```python
from build123d import *

# Parameters (mm, degrees)
BOSS_EXTRUDE1_DEPTH = 11
CUT_EXTRUDE1_DEPTH  = 7
SKETCH4_R           = 1.6
CUT_EXTRUDE2_DEPTH  = 19.607794066
SKETCH5_R           = 1.25
CUT_EXTRUDE3_DEPTH  = 21.451161336
CUT_EXTRUDE4_DEPTH  = 21.451161336
CUT_EXTRUDE5_DEPTH  = 5.8
SKETCH9_W           = 6.962435565
SKETCH9_H           = 4.2
CUT_EXTRUDE6_DEPTH  = 5.8
BOSS_EXTRUDE3_START = 0.2
BOSS_EXTRUDE3_DEPTH = 0.2
BOSS_EXTRUDE4_DEPTH = 7.3
CUT_EXTRUDE7_DEPTH  = 1.6


with BuildPart() as part:
    # Sketch1 → Boss-Extrude1 (new body)
    with BuildSketch(Plane.XY):
        Polygon((-8.5, 0), (8.5, 0), (8.5, 9), (7.5, 9), (7.5, 15), (-7.5, 15), (-7.5, 9), (-8.5, 9), align=None)
    extrude(amount=BOSS_EXTRUDE1_DEPTH)

    # Sketch2 → Cut-Extrude1 (cut)
    with BuildSketch(Plane.XY.offset(11)):
        with BuildLine():
            Line((3, 18), (3, 12))
            ThreePointArc((3, 12), (0, 9), (-3, 12))
            Line((-3, 12), (-3, 18))
            ThreePointArc((-3, 18), (0, 21), (3, 18))
        make_face()
    extrude(amount=-CUT_EXTRUDE1_DEPTH, mode=Mode.SUBTRACT)

    # Sketch4 → Cut-Extrude2 (cut, through all)
    with BuildSketch(Plane.XY.offset(4)):
        with Locations((0, 12)):
            Circle(SKETCH4_R)
    extrude(amount=-CUT_EXTRUDE2_DEPTH, mode=Mode.SUBTRACT)

    # Sketch5 → Cut-Extrude3 (cut, through all)
    with BuildSketch(Plane.XY.offset(11)):
        with Locations((-4.75, 4.5)):
            Circle(SKETCH5_R)
        with Locations(Location((4.75, 4.5, 0), (0, 0, 180))):
            Circle(SKETCH5_R)
    extrude(amount=-CUT_EXTRUDE3_DEPTH, mode=Mode.SUBTRACT)

    # Sketch7 → Cut-Extrude4 (cut, through all)
    with BuildSketch(Plane.XY.offset(11)):
        with BuildLine():
            Line((-6.75, 5.75), (-2.75, 5.75))
            ThreePointArc((-2.75, 5.75), (-1.5, 4.5), (-2.75, 3.25))
            Line((-2.75, 3.25), (-6.75, 3.25))
            ThreePointArc((-6.75, 3.25), (-8, 4.5), (-6.75, 5.75))
        make_face()
        with BuildLine():
            Line((6.75, 3.25), (2.75, 3.25))
            ThreePointArc((2.75, 3.25), (1.5, 4.5), (2.75, 5.75))
            Line((2.75, 5.75), (6.75, 5.75))
            ThreePointArc((6.75, 5.75), (8, 4.5), (6.75, 3.25))
        make_face()
    extrude(amount=-CUT_EXTRUDE4_DEPTH, mode=Mode.SUBTRACT)

    # Sketch8 → Cut-Extrude5 (cut)
    with BuildSketch(Plane(origin=(0, 0, 0), x_dir=(-1, 0, 0), z_dir=(0, 0, -1))):
        Polygon((-1.537564435, 6.6), (-3.962435565, 6.6), (-5.174871131, 4.5), (-3.962435565, 2.4), (-1.537564435, 2.4), (-0.325128869, 4.5), align=None)
        Polygon((1.537564435, 6.6), (0.325128869, 4.5), (1.537564435, 2.4), (3.962435565, 2.4), (5.174871131, 4.5), (3.962435565, 6.6), align=None)
    extrude(amount=-CUT_EXTRUDE5_DEPTH, mode=Mode.SUBTRACT)

    # Sketch9 → Cut-Extrude6 (cut)
    with BuildSketch(Plane(origin=(0, 0, 5.8), x_dir=(-1, 0, 0), z_dir=(0, 0, -1))):
        with Locations((5.018782218, 4.5)):
            Rectangle(SKETCH9_W, SKETCH9_H)
        with Locations((-5.018782218, 4.5)):
            Rectangle(SKETCH9_W, SKETCH9_H)
    extrude(amount=CUT_EXTRUDE6_DEPTH, mode=Mode.SUBTRACT)

    # Sketch11 → Boss-Extrude3 (add)
    with BuildSketch(Plane.XY.offset(4).offset(BOSS_EXTRUDE3_START)):
        with BuildLine():
            Line((3, 15), (-3, 15))
            Line((-3, 15), (-3, 12))
            ThreePointArc((-3, 12), (0, 9), (3, 12))
            Line((3, 12), (3, 15))
        make_face()
    extrude(amount=-BOSS_EXTRUDE3_DEPTH)

    # Sketch12 → Boss-Extrude4 (add)
    with BuildSketch(Plane(origin=(0, 0, 5.8), x_dir=(-1, 0, 0), z_dir=(0, 0, -1))):
        with BuildLine():
            Line((1.5, 8.9), (1.5, 6.936860279))
            ThreePointArc((1.5, 6.936860279), (0, 5.436860279), (-1.5, 6.936860279))
            Line((-1.5, 6.936860279), (-1.5, 8.9))
            ThreePointArc((-1.5, 8.9), (0, 10.4), (1.5, 8.9))
        make_face()
        with BuildLine():
            Line((1.5, 2.063139721), (1.5, 1.5))
            ThreePointArc((1.5, 1.5), (0, 0), (-1.5, 1.5))
            Line((-1.5, 1.5), (-1.5, 2.063139721))
            ThreePointArc((-1.5, 2.063139721), (0, 3.563139721), (1.5, 2.063139721))
        make_face()
    extrude(amount=BOSS_EXTRUDE4_DEPTH)

    # Sketch13 → Cut-Extrude7 (cut)
    with BuildSketch(Plane.XY.offset(5.8)):
        with BuildLine():
            ThreePointArc((1.42730909, 9.361290323), (0, 10.4), (-1.42730909, 9.361290323))
            ThreePointArc((-1.42730909, 9.361290323), (0, 9), (1.42730909, 9.361290323))
        make_face()
    extrude(amount=-CUT_EXTRUDE7_DEPTH, mode=Mode.SUBTRACT)


solid = part.part
```
Geometry: final body of the model. Coordinates: model frame, mm. A direction names the side the tool comes from. Coordinates: 2 decimals unless noted, no trailing zeros. Order: outer loops, then holes, each group sorted by start corner. A loop starts at its lowest first (then second) coordinate and runs counter-clockwise, first axis right, second up. Notation, with made-up numbers: (-11, 42) - (6, 42) arc R20 ccw to (6, 61) - close; hole circle Ø5 at (-34.5, 17.5). An arc over 180 degrees is marked (long way). Write each question's results on one line, items separated by ' | '.
(1) Section query C-C, the plane y = 12.5. Return the cut outline in (x, z).
Values found:
outline: (-7.5, 0) - (-1.52, 0) - (-1.52, 4) - (1.52, 4) - (1.52, 0) - (7.5, 0) - (7.5, 11) - (3, 11) - (3, 4.2) - (-3, 4.2) - (-3, 11) - (-7.5, 11) - close
(2) Section query B-B, the plane z = 0.5. Return the cut outline in (x, y), plus the area to 3 significant figures.
Values found:
outline: (-8.5, 0) - (8.5, 0) - (8.5, 2.4) - (1.54, 2.4) - (0.33, 4.5) - (1.54, 6.6) - (8.5, 6.6) - (8.5, 9) - (7.5, 9) - (7.5, 15) - (-7.5, 15) - (-7.5, 9) - (-8.5, 9) - (-8.5, 6.6) - (-1.54, 6.6) - (-0.33, 4.5) - (-1.54, 2.4) - (-8.5, 2.4) - close; hole circle Ø3.2 at (0, 12) | area: 171 mm²
(3) Mould query, pull axis Y, two halves, no side actions, for faces 1 (the face through (1.5, 8, -1)), 2 (the face through (0, 0, -1)), 3 (the face through (0.94, 3.435, 2.859)), 4 (the face through (5, 2.4, 3)). Classes: +Y half, -Y half, draft (parallel to the pull), parting line (faces both ways), or undercut.
Values found:
face 1: draft | face 2: -Y half | face 3: undercut | face 4: undercut
(4) Line query: line 1 (X direction, y = 12, z = 0.9); line 2 (Y direction, x = -4, z = 7.75); line 3 (Y direction, x = 3.5, z = 2.25). Output: solid intervals per line, ascending. Write a range as [from, to].
Values found:
line 1: x = [-7.5, -1.6], [1.6, 7.5] | line 2: y = [0, 3.25], [5.75, 15] | line 3: y = [0, 2.4], [6.6, 15]
(5) First-contact query: pin 1 Ø3.5 at (x, y) = (-4, 4) entering from -Z; pin 2 Ø3 at (x, y) = (1, 12) entering from +Z; pin 3 Ø6.5 at (x, z) = (-5.5, 3.5) entering from -Y; pin 4 Ø3 at (y, z) = (13, 4.5) entering from -X. Flat tips, straight axial feed; report the tip coordinate or a pass-through.
Values found:
pin 1: stops at z = 0 | pin 2: stops at z = 4.2 | pin 3: stops at y = 0 | pin 4: stops at x = -7.5
(6) Section query A-A, the plane x = -3.75. Return the cut outline in (y, z), plus the area to 3 significant figures.
Values found:
outline: (0, 0) - (2.4, 0) - (2.4, 5.8) - (3.25, 5.8) - (3.25, 11) - (0, 11) - close; (5.75, 5.8) - (6.6, 5.8) - (6.6, 0) - (15, 0) - (15, 11) - (5.75, 11) - close | area: 128 mm²
(7) Set-up query: faces 5 (the face through (-0.208, 13.586, 2.028)), 6 (the face through (0, 9, 8)), 7 (the face through (-1.5, 8, -1)), 8 (the face through (1.5, 4.5, 8.4)). Return all of +Z, -Z, +X, -X, +Y, -Y with unobstructed straight access to the full face (end or side cutting, diameter ignored); none if empty.
Values found:
face 5: -Z | face 6: +Z, +Y | face 7: -Z, -X, +Y, -Y | face 8: +Z, -Z
